from build123d import *

# Parameters (mm, degrees)
SKETCH1_W           = 45
SKETCH1_H           = 140
SKETCH1_H_2         = 45
SKETCH1_W_2         = 260
BOSS_EXTRUDE1_DEPTH = 12.5
SKETCH2_R           = 2
CUT_EXTRUDE1_DEPTH  = 15
SKETCH3_R           = 2
CUT_EXTRUDE2_DEPTH  = 15


with BuildPart() as part:
    # Sketch1 → Boss-Extrude1 (new body)
    with BuildSketch(Plane.XY):
        Polygon((200, 0), (0, 0), (-200, 0), (-200, -222.5), (-154.126087164, -274.927328955), (-130, -274.927328955), (-130, -222.5), (130, -222.5), (130, -274.927328955), (154.126087164, -274.927328955), (200, -222.5), align=None)
        Polygon((-142.5, -267.654601682), (-182.010276472, -222.5), (-142.5, -222.5), align=None, mode=Mode.SUBTRACT)
        Polygon((142.5, -222.5), (182.010276472, -222.5), (142.5, -267.654601682), align=None, mode=Mode.SUBTRACT)
        with Locations((-165, -140)):
            Rectangle(SKETCH1_W, SKETCH1_H, mode=Mode.SUBTRACT)
        with Locations((-165, -35)):
            Rectangle(SKETCH1_W, SKETCH1_H_2, mode=Mode.SUBTRACT)
        with Locations((0, -35)):
            Rectangle(SKETCH1_W_2, SKETCH1_H_2, mode=Mode.SUBTRACT)
        with Locations((0, -140)):
            Rectangle(SKETCH1_W_2, SKETCH1_H, mode=Mode.SUBTRACT)
        with Locations((165, -140)):
            Rectangle(SKETCH1_W, SKETCH1_H, mode=Mode.SUBTRACT)
        with Locations((165, -35)):
            Rectangle(SKETCH1_W, SKETCH1_H_2, mode=Mode.SUBTRACT)
    extrude(amount=BOSS_EXTRUDE1_DEPTH)

    # Sketch2 → Cut-Extrude1 (cut)
    with BuildSketch(Plane(origin=(0, 0, 0), x_dir=(-1, 0, 0), z_dir=(0, 0, -1))):
        with Locations((136.25, -110)):
            Circle(SKETCH2_R)
        with Locations((136.25, -150)):
            Circle(SKETCH2_R)
        with Locations((-136.25, -110)):
            Circle(SKETCH2_R)
        with Locations((-136.25, -150)):
            Circle(SKETCH2_R)
    extrude(amount=-CUT_EXTRUDE1_DEPTH, mode=Mode.SUBTRACT)

    # Sketch3 → Cut-Extrude2 (cut)
    with BuildSketch(Plane.XY.offset(12.5)):
        with Locations((-136.25, -237.927328955)):
            Circle(SKETCH3_R)
        with Locations((-136.25, -254.927328955)):
            Circle(SKETCH3_R)
        with Locations((136.25, -254.927328955)):
            Circle(SKETCH3_R)
        with Locations((136.25, -237.927328955)):
            Circle(SKETCH3_R)
    extrude(amount=-CUT_EXTRUDE2_DEPTH, mode=Mode.SUBTRACT)


solid = part.part
Check sheet for the modelled part. Datum: model origin and axes. Units: mm. A direction names the side the tool comes from. Round coordinates to 2 decimals unless told otherwise and drop trailing zeros. Order: outer loops, then holes, each group sorted by start corner. A loop starts at its lowest first (then second) coordinate and runs counter-clockwise, first axis right, second up.
(1) Access from +Z, -Z, +X, -X, +Y, -Y to the whole of each face (thin tool, end or side, straight path). Record for faces 4 (the flat face through (-2, -222.5, 6)), 5 (the flat face through (-2, -70, 6)).
(2) Draft check along X on faces 1 (the flat face through (165, -57.5, 6)), 2 (the flat face through (-16, -66, 12.5)), 3 (the flat face through (200, -113, 6)). Enter one of: pulls with the +X half, pulls with the -X half, needs draft (parallel to the pull), parting line crosses it, or undercut.
(3) Cross-section at A-A, the plane y = -41. Enter the section's corners in (x, z).
(4) Cross-section at C-C, the plane z = 9. State how many separate pieces and enclosed holes the cut face has, and give its area (3 significant figures).
(5) Go/stop test with flat-tipped pins: P1, Ø2, axis at x = -3, z = 7.5, coming from the -Y side; P2, Ø12, axis at x = -54, y = -231, coming from the -Z side. Record where each tip stops, or that it passes through.
(6) Scan lines: probe 1 along X at (y, z) = (-37.5, 9); probe 2 along Y at (x, z) = (-136.25, 8.75); probe 3 along Y at (x, z) = (84, 0.75). Record each from-to range of solid material in increasing order.
(7) Cross-section at B-B, the plane x = -169. Enter the section's corners in (y, z).
Check sheet entries:
1. face 4: +Z, -Z, -Y
1. face 5: +Z, -Z
2. face 1: undercut
2. face 2: needs draft
2. face 3: pulls with the +X half
3. outline: (-200, 0) - (-187.5, 0) - (-187.5, 12.5) - (-200, 12.5) - close; (-142.5, 0) - (-130, 0) - (-130, 12.5) - (-142.5, 12.5) - close; (130, 0) - (142.5, 0) - (142.5, 12.5) - (130, 12.5) - close; (187.5, 0) - (200, 0) - (200, 12.5) - (187.5, 12.5) - close
4. separate pieces: 1
4. enclosed holes: 16
4. area: 27,300 mm2
5. P1: stops at y = -222.5
5. P2: passes through
6. probe 1: x = -200 to -187.5, -142.5 to -130, 130 to 142.5, 187.5 to 200
6. probe 2: y = -274.93 to -256.93, -252.93 to -239.93, -235.93 to -152, -148 to -112, -108 to 0
6. probe 3: y = -222.5 to -210, -70 to -57.5, -12.5 to 0
7. outline: (-257.93, 0) - (-237.37, 0) - (-237.37, 12.5) - (-257.93, 12.5) - close; (-222.5, 0) - (-210, 0) - (-210, 12.5) - (-222.5, 12.5) - close; (-70, 0) - (-57.5, 0) - (-57.5, 12.5) - (-70, 12.5) - close; (-12.5, 0) - (0, 0) - (0, 12.5) - (-12.5, 12.5) - close
